CAD build for the part. Positions are in the model's coordinates, mm. Round coordinates to 2 decimals unless told otherwise and drop trailing zeros. Loops run counter-clockwise (first coordinate to the right, second up) from the corner with the lowest first, then second, coordinate; pieces in that order, holes last.
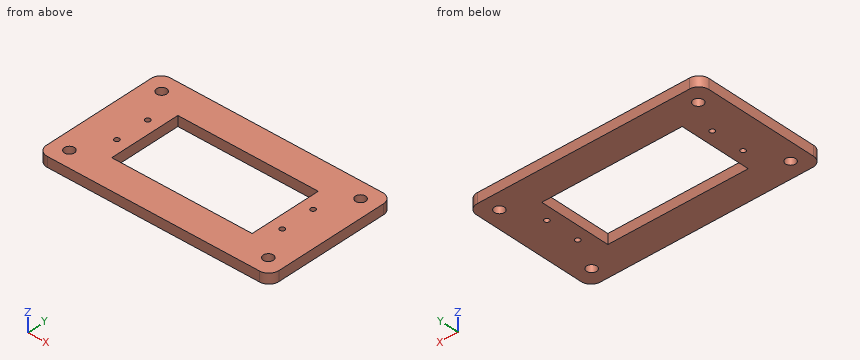
from build123d import *

# Parameters (mm, degrees)
F0_W     = 69.5
F0_H     = 40
F0_R     = 1.5
F0_R_2   = 0.75
F0_W_2   = 42
F0_H_2   = 21.5
F1_DEPTH = 3
F2_R     = 3


with BuildPart() as f1:
    # F0 (on Top) → F1 (new body)
    with BuildSketch(Plane.XY):
        Rectangle(F0_W, F0_H)
        with Locations((-29.75, -15)):
            Circle(F0_R, mode=Mode.SUBTRACT)
        with Locations((-24.75, -5)):
            Circle(F0_R_2, mode=Mode.SUBTRACT)
        with Locations((29.75, -15)):
            Circle(F0_R, mode=Mode.SUBTRACT)
        with Locations((24.75, -5)):
            Circle(F0_R_2, mode=Mode.SUBTRACT)
        with Locations((-24.75, 5)):
            Circle(F0_R_2, mode=Mode.SUBTRACT)
        with Locations((-29.75, 15)):
            Circle(F0_R, mode=Mode.SUBTRACT)
        Rectangle(F0_W_2, F0_H_2, mode=Mode.SUBTRACT)
        with Locations((24.75, 5)):
            Circle(F0_R_2, mode=Mode.SUBTRACT)
        with Locations((29.75, 15)):
            Circle(F0_R, mode=Mode.SUBTRACT)
    extrude(amount=F1_DEPTH)

    # F2
    f2_edges = [f1.edges().sort_by_distance(p)[0] for p in [
        (-34.75, -20, 1.5),
        (34.75, -20, 1.5),
        (34.75, 20, 1.5),
        (-34.75, 20, 1.5),
    ]]
    fillet(f2_edges, radius=F2_R)


solid = f1.part
Item 1: Cut at D-D (z = 1.7). State how many separate pieces and enclosed holes the cut face has, plus the area to 3 significant figures.
Verdict:
separate pieces: 1
enclosed holes: 9
area: 1,830 mm2
Item 2: Cut at B-B (x = -29.75). List the corners of the cut face in (y, z).
Verdict:
outline: (-20, 0) - (-16.5, 0) - (-16.5, 3) - (-20, 3) - close; (-13.5, 0) - (13.5, 0) - (13.5, 3) - (-13.5, 3) - close; (16.5, 0) - (20, 0) - (20, 3) - (16.5, 3) - close
Item 3: Cut at A-A (y = -5). List the corners of the cut face in (x, z), plus the area to 3 significant figures.
Verdict:
outline: (-34.75, 0) - (-25.5, 0) - (-25.5, 3) - (-34.75, 3) - close; (-24, 0) - (-21, 0) - (-21, 3) - (-24, 3) - close; (21, 0) - (24, 0) - (24, 3) - (21, 3) - close; (25.5, 0) - (34.75, 0) - (34.75, 3) - (25.5, 3) - close
area: 73.5 mm2
Item 4: Cut at C-C (y = 3.5). List the corners of the cut face in (x, z).
Verdict:
outline: (-34.75, 0) - (-21, 0) - (-21, 3) - (-34.75, 3) - close; (21, 0) - (34.75, 0) - (34.75, 3) - (21, 3) - close
Item 5: Flat gauge pin, fed straight in: P1, Ø5, axis at x = -29.75, y = 15, coming from the -Z side. Where does the tip first touch, or does it go through?
Verdict:
P1: stops at z = 0
Item 6: Wall check: L1, parallel to X at y = 6, z = 1.65; L2, parallel to Y at x = -30.5, z = 0.4; L3, parallel to Y at x = -24.75, z = 2.25. Give the ranges that are in metal, low to high.
Verdict:
L1: x = -34.75 to -21, 21 to 34.75
L2: y = -20 to -16.3, -13.7 to 13.7, 16.3 to 20
L3: y = -20 to -5.75, -4.25 to 4.25, 5.75 to 20
